Part model, mm, in its own coordinate system. Face numbers are marked on the shaded views. A direction names the side the tool comes from. Round coordinates to 2 decimals unless told otherwise and drop trailing zeros. Loops run counter-clockwise (first coordinate to the right, second up) from the corner with the lowest first, then second, coordinate; pieces in that order, holes last. Notation, with made-up numbers: (89.5, 56) -> (94.5, 56) arc R19 cw to (94.5, 68) -> close; hole circle Ø10 at (64, 27.5). An arc over 180 degrees is marked (long way). Use a Markdown table: item, result. Add a question column.
Item 1: Probe line 1 (X direction, y = 11.25, z = 32.5); line 2 (Z direction, x = 16, y = 11.25); line 3 (Z direction, x = -16.5, y = 9.75). List the from-to ranges inside material, lowest first. Write a range as [from, to].
Item 2: Cut at B-B, the plane z = 13.5. List the corners of the cut face in (x, y), plus the area to 3 significant figures.
Item 3: Which spindle directions (+Z, -Z, +X, -X, +Y, -Y) get a long thin tool onto all of the face, cutting with end or side? Do the marked faces 1, 2 and 3. Say none if no direction does.
Item 4: Cut at C-C, the plane y = 4.5. List the corners of the cut face in (x, z), plus the area to 3 significant figures.
Item 5: Flat gauge pins, fed straight in: pin 1 (6 mm diameter, centred on x = -6, y = 3.5, fed in from -Z); pin 2 (5 mm diameter, centred on y = 6, z = 34, fed in from +X); pin 3 (14 mm diameter, centred on x = 4.5, z = 28.5, fed in from +Y) (3 decimals). Where does each tip first touch, or does it go through?
Item 6: Cut at A-A, the plane x = 0. List the corners of the cut face in (y, z) (3 decimals), plus the area to 3 significant figures.
Item 7: Two-plate mould, pull along X, no slides. Class the marked faces 4, 5 and 6: pulls with the +X half, pulls with the -X half, needs draft (parallel to the pull), parting line crosses it, or undercut.
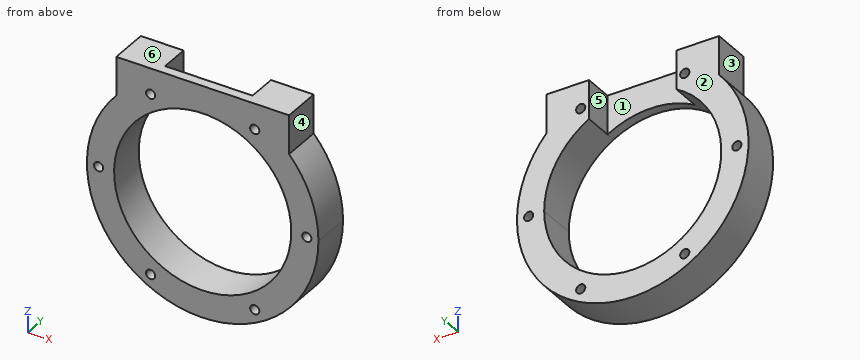
```python
from build123d import *
from build123d.topology import SkipClean

# Parameters (mm, degrees)
BOSS_EXTRUDE1_DEPTH   = 12.7
SKETCH5_W             = 13.961436905
SKETCH5_H             = 12.7
BOSS_EXTRUDE3_DEPTH   = 12.7
F_3_0MM_DOWEL_HOLE1_D = 3
BOSS_EXTRUDE4_DEPTH   = 3.175


with BuildPart() as part:
    # Sketch1 → Boss-Extrude1 (new body)
    with BuildSketch(Plane(origin=(0, 0, 0), x_dir=(1, 0, 0), z_dir=(0, 1, 0))):
        with BuildLine():
            ThreePointArc((28.956, 0), (25.021578547, -14.572938722), (14.2875, -25.18565623))
            Line((14.2875, -25.18565623), (28.248936905, -25.18565623))
            ThreePointArc((28.248936905, -25.18565623), (35.365442045, -13.476098284), (37.846, 0))
            ThreePointArc((37.846, 0), (-13.476098284, 35.365442045), (-28.248936905, -25.18565623))
            Line((-28.248936905, -25.18565623), (-14.2875, -25.18565623))
            ThreePointArc((-14.2875, -25.18565623), (-14.572938722, 25.021578547), (28.956, 0))
        make_face()
    extrude(amount=BOSS_EXTRUDE1_DEPTH)

    # Sketch5 → Boss-Extrude3 (add)
    with BuildSketch(Plane.XY.offset(25.18565623)):
        with Locations((-21.268218453, 6.35)):
            Rectangle(SKETCH5_W, SKETCH5_H)
        with Locations((21.268218453, 6.35)):
            Rectangle(SKETCH5_W, SKETCH5_H)
    extrude(amount=BOSS_EXTRUDE3_DEPTH)

    # Ø3.0mm Dowel Hole1 (through all)
    with Locations(Plane(origin=(0, 0, 0), x_dir=(-1, 0, 0), z_dir=(0, -1, 0))):
        with Locations((-17.018, 29.476040643), (-34.036, 0), (17.018, 29.476040643), (34.036, 0), (17.018, -29.476040643), (-17.018, -29.476040643)):
            Hole(F_3_0MM_DOWEL_HOLE1_D / 2)

    # Sketch11 → Boss-Extrude4 (add)
    with SkipClean():  # the faces are left unmerged after this step: merging them gives an invalid solid
        with BuildSketch(Plane.XZ):
            with BuildLine():
                ThreePointArc((-14.2875, 25.18565623), (0, 28.956), (14.2875, 25.18565623))
                Line((14.2875, 25.18565623), (14.2875, 37.88565623))
                Line((14.2875, 37.88565623), (-14.2875, 37.88565623))
                Line((-14.2875, 37.88565623), (-14.2875, 25.18565623))
            make_face()
        extrude(amount=-BOSS_EXTRUDE4_DEPTH)


solid = part.part
```
A:
| question | item | result |
|---|---|---|
| 1 | line 1 | x = [-28.25, -14.29], [14.29, 28.25] |
| 1 | line 2 | z = [-34.3, -30.58], [-28.37, -24.13], [24.13, 28.37], [30.58, 37.89] |
| 1 | line 3 | z = [-34.06, -30.88], [-28.07, -23.79], [23.79, 28.07], [30.88, 37.89] |
| 2 | outline | (-35.36, 0) -> (-25.62, 0) -> (-25.62, 12.7) -> (-35.36, 12.7) -> close; (25.62, 0) -> (35.36, 0) -> (35.36, 12.7) -> (25.62, 12.7) -> close |
| 2 | area | 247 mm^2 |
| 3 | face 1 | +Z, +Y |
| 3 | face 2 | +Z, -Z, +X, -X, +Y |
| 3 | face 3 | +Z, -X, +Y, -Y |
| 4 | outline | (-28.25, 25.19) arc R37.85 ccw (long way) to (28.25, 25.19) -> (28.25, 37.89) -> (14.29, 37.89) -> (14.29, 25.19) arc R28.96 cw (long way) to (-14.29, 25.19) -> (-14.29, 37.89) -> (-28.25, 37.89) -> close; hole circle Ø3 at (-34.04, 0); hole circle Ø3 at (-17.02, -29.48); hole circle Ø3 at (-17.02, 29.48); hole circle Ø3 at (17.02, -29.48); hole circle Ø3 at (17.02, 29.48); hole circle Ø3 at (34.04, 0) |
| 4 | area | 1,760 mm^2 |
| 5 | pin 1 | stops at z = -37.73 |
| 5 | pin 2 | stops at x = 28.25 |
| 5 | pin 3 | stops at y = 3.175 |
| 6 | outline | (0, -37.846) -> (12.7, -37.846) -> (12.7, -28.956) -> (0, -28.956) -> close; (0, 28.956) -> (3.175, 28.956) -> (3.175, 37.886) -> (0, 37.886) -> close |
| 6 | area | 141 mm^2 |
| 7 | face 4 | pulls with the +X half |
| 7 | face 5 | undercut |
| 7 | face 6 | needs draft |
